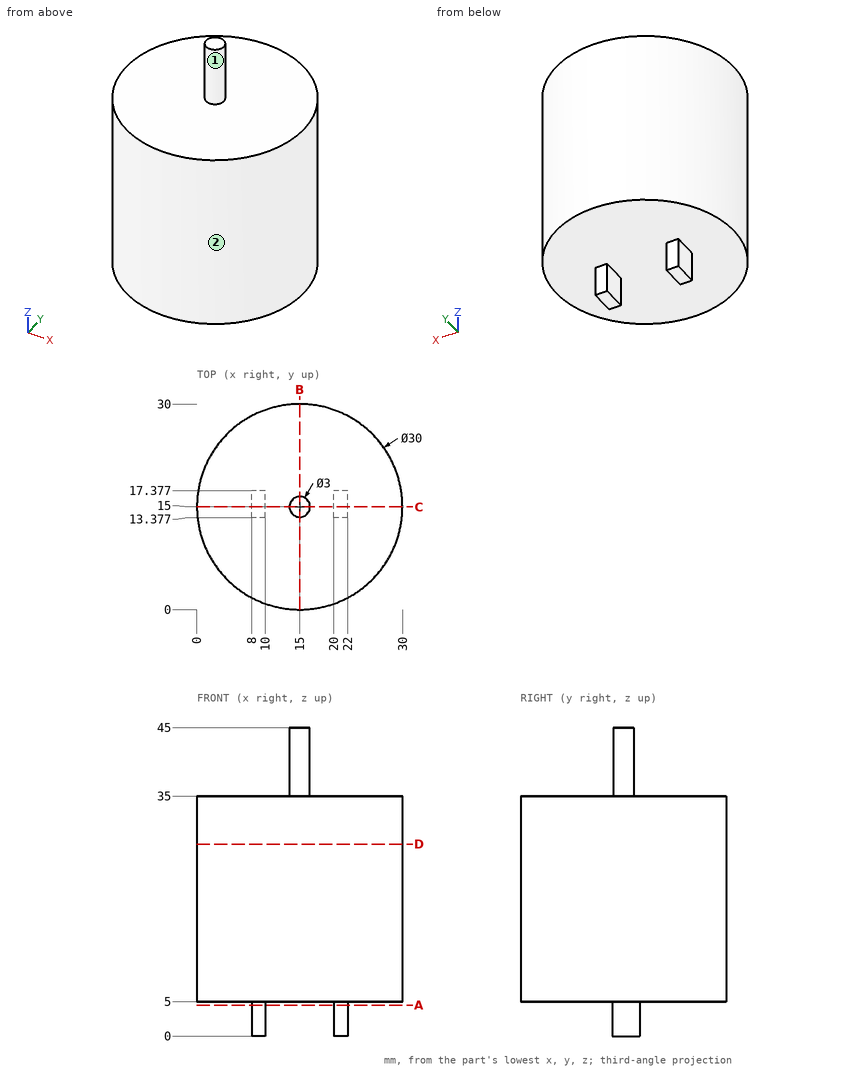
Check sheet for the drawn part. Datum: minimum x, y, z corner. Units: mm. A direction names the side the tool comes from. Give positions to 0.01 mm unless a question says otherwise; leave off trailing zeros. Order: outer loops, then holes, each group sorted by start corner. A loop starts at its lowest first (then second) coordinate and runs counter-clockwise, first axis right, second up. Notation, with made-up numbers: (86, -23) -> (99, -23) arc R16 cw to (99, -12) -> close; hole circle Ø4 at (13.25, 47). An arc over 180 degrees is marked (long way). Use a Markdown table: item, result.
1) Section check C-C, the plane y = 15. Record the boundary of the cut face in (x, z), then the cut area to 3 significant figures.
Results:
| item | result |
|---|---|
| outline | (0, 5) -> (8, 5) -> (8, 0) -> (10, 0) -> (10, 5) -> (20, 5) -> (20, 0) -> (22, 0) -> (22, 5) -> (30, 5) -> (30, 35) -> (16.5, 35) -> (16.5, 45) -> (13.5, 45) -> (13.5, 35) -> (0, 35) -> close |
| area | 950 mm² |
2) Section check B-B, the plane x = 15. Record the boundary of the cut face in (y, z), then the cut area to 3 significant figures.
Results:
| item | result |
|---|---|
| outline | (0, 5) -> (30, 5) -> (30, 35) -> (16.5, 35) -> (16.5, 45) -> (13.5, 45) -> (13.5, 35) -> (0, 35) -> close |
| area | 930 mm² |
3) Section check D-D, the plane z = 28. Record the boundary of the cut face in (x, y).
Results:
| item | result |
|---|---|
| outline | circle Ø30 at (15, 15) |
4) Section check A-A, the plane z = 4.5. Record the boundary of the cut face in (x, y), then the cut area to 3 significant figures.
Results:
| item | result |
|---|---|
| outline | (8, 13.38) -> (10, 13.38) -> (10, 17.38) -> (8, 17.38) -> close; (20, 13.38) -> (22, 13.38) -> (22, 17.38) -> (20, 17.38) -> close |
| area | 16.0 mm² |
5) Tool access check on the marked faces 1 and 2. Record the directions out of +Z, -Z, +X, -X, +Y, -Y that give a thin tool (end or side, any length) a straight path to the whole face; none if there is none.
Results:
| item | result |
|---|---|
| face 1 | +Z |
| face 2 | +Z, -Z |
6) Material ranges on probe 1 along X at (y, z) = (14.75, 14); probe 2 along Z at (x, y) = (19, 17.5); probe 3 along Z at (x, y) = (9.5, 13.75), recorded low to high.
Results:
| item | result |
|---|---|
| probe 1 | 0 to 30 |
| probe 2 | 5 to 35 |
| probe 3 | 0 to 35 |
7) Depth check by flat-ended pin: pin 1 Ø1.5 at (y, z) = (16, 39) entering from -X; pin 2 Ø8 at (x, y) = (25.5, 6) entering from +Z; pin 3 Ø1 at (x, y) = (18.5, 15.5) entering from -Z; pin 4 Ø12 at (y, z) = (13.5, 17) entering from -X. Enter the tip coordinate at first touch or a pass-through.
Results:
| item | result |
|---|---|
| pin 1 | x = 13.52 |
| pin 2 | z = 35 |
| pin 3 | z = 5 |
| pin 4 | x = 0 |
